Geometry check sheet. Reference: the model listing, model coordinates, mm. Face numbers are marked on the shaded views. A direction names the side the tool comes from. Give positions to 0.01 mm unless a question says otherwise; leave off trailing zeros. Order: outer loops, then holes, each group sorted by start corner. A loop starts at its lowest first (then second) coordinate and runs counter-clockwise, first axis right, second up. Notation, with made-up numbers: M -8,32.5 L 10,32.5 A23 cw 10,48.5 Z; hole C 30,21 d5. An arc over 180 degrees is marked long. Answer as CSV lines item,"result".
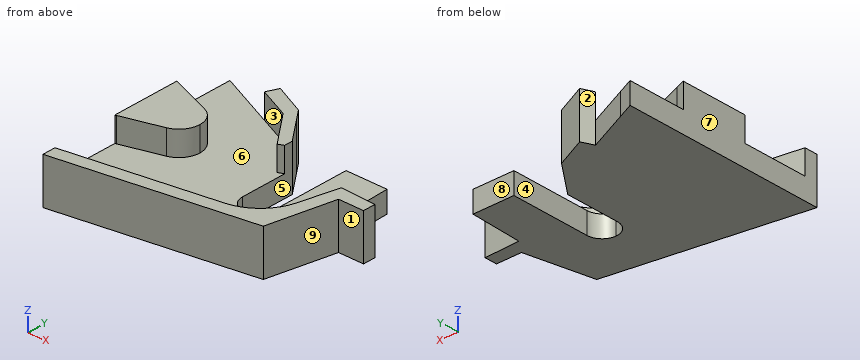
from build123d import *

# Parameters (mm, degrees)
BOSS_EXTRUDE2_DEPTH = 7
BOSS_EXTRUDE3_DEPTH = 15


with BuildPart() as part:
    # Sketch1 → Boss-Extrude2 (new body)
    with BuildSketch(Plane.XY):
        with BuildLine():
            Line((-40.950735345, 0.950710087), (-41.446212302, -3.10814846))
            Line((-41.446212302, -3.10814846), (-41.446212302, -20.792174742))
            Line((-41.446212302, -20.792174742), (-1.475395331, -14.281320254))
            Line((-1.475395331, -14.281320254), (6.869125611, -12.922079544))
            ThreePointArc((6.869125611, -12.922079544), (-10.497186211, -1.975719261), (-2.67291579, 17.003015737))
            Line((-2.67291579, 17.003015737), (-11.698348753, 29.052034329))
            Line((-11.698348753, 29.052034329), (-22.155090004, 33.745741812))
            Line((-22.155090004, 33.745741812), (-36.178915637, 40.040603064))
            Line((-36.178915637, 40.040603064), (-38.38035072, 22.006840878))
            Line((-38.38035072, 22.006840878), (-27.430483413, 17.813364482))
            ThreePointArc((-27.430483413, 17.813364482), (-24.205719333, 15.274219005), (-22.987821209, 11.354641568))
            ThreePointArc((-22.987821209, 11.354641568), (-24.378521993, 7.195004916), (-27.991340604, 4.708206285))
            Line((-27.991340604, 4.708206285), (-40.950735345, 0.950710087))
        make_face()
        Polygon((-41.446212302, 23.180975488), (-38.38035072, 22.006840878), (-36.178915637, 40.040603064), (-41.446212302, 42.4049295), align=None)
        with BuildLine():
            Line((-38.38035072, 22.006840878), (-40.950735345, 0.950710087))
            Line((-40.950735345, 0.950710087), (-27.991340604, 4.708206285))
            ThreePointArc((-27.991340604, 4.708206285), (-30.199701974, 4.44480386), (-32.377484382, 4.895918653))
            ThreePointArc((-32.377484382, 4.895918653), (-36.813821606, 11.650359644), (-31.816627191, 18.00107685))
            ThreePointArc((-31.816627191, 18.00107685), (-29.608265822, 18.264479276), (-27.430483413, 17.813364482))
            Line((-27.430483413, 17.813364482), (-38.38035072, 22.006840878))
        make_face()
        Polygon((-41.446212302, 0.807049614), (-40.950735345, 0.950710087), (-38.38035072, 22.006840878), (-41.446212302, 23.180975488), align=None)
        with BuildLine():
            Line((-32.377484382, 4.895918653), (-29.903983898, 11.354641568))
            Line((-29.903983898, 11.354641568), (-31.816627191, 18.00107685))
            ThreePointArc((-31.816627191, 18.00107685), (-36.813821606, 11.650359644), (-32.377484382, 4.895918653))
        make_face()
        with BuildLine():
            Line((-29.903983898, 11.354641568), (-27.430483413, 17.813364482))
            ThreePointArc((-27.430483413, 17.813364482), (-29.608265822, 18.264479276), (-31.816627191, 18.00107685))
            Line((-31.816627191, 18.00107685), (-29.903983898, 11.354641568))
        make_face()
        with BuildLine():
            ThreePointArc((-32.377484382, 4.895918653), (-30.199701974, 4.44480386), (-27.991340604, 4.708206285))
            Line((-27.991340604, 4.708206285), (-29.903983898, 11.354641568))
            Line((-29.903983898, 11.354641568), (-32.377484382, 4.895918653))
        make_face()
        with BuildLine():
            Line((-29.903983898, 11.354641568), (-27.991340604, 4.708206285))
            ThreePointArc((-27.991340604, 4.708206285), (-24.378521993, 7.195004916), (-22.987821209, 11.354641568))
            ThreePointArc((-22.987821209, 11.354641568), (-24.205719333, 15.274219005), (-27.430483413, 17.813364482))
            Line((-27.430483413, 17.813364482), (-29.903983898, 11.354641568))
        make_face()
        with BuildLine():
            Line((-41.446212302, -20.792174742), (-41.446212302, -25.123400981))
            Line((-41.446212302, -25.123400981), (21.822672825, -14.817519442))
            Line((21.822672825, -14.817519442), (26.489801196, 7.266810726))
            Line((26.489801196, 7.266810726), (34.744303123, 7.266810726))
            Line((34.744303123, 7.266810726), (34.744303123, 11.354641566))
            Line((34.744303123, 11.354641566), (23.2245968, 11.838054321))
            Line((23.2245968, 11.838054321), (20.289273371, -0.393165966))
            ThreePointArc((20.289273371, -0.393165966), (20.186058412, -0.853126065), (20.069286081, -1.309832583))
            ThreePointArc((20.069286081, -1.309832583), (15.501382573, -8.842559665), (7.629856976, -12.798163857))
            ThreePointArc((7.629856976, -12.798163857), (7.250240456, -12.864720887), (6.869125611, -12.922079544))
            Line((6.869125611, -12.922079544), (-1.475395331, -14.281320254))
            Line((-1.475395331, -14.281320254), (-41.446212302, -20.792174742))
        make_face()
        with BuildLine():
            ThreePointArc((-2.67291579, 17.003015737), (-10.497186211, -1.975719261), (6.869125611, -12.922079544))
            Line((6.869125611, -12.922079544), (7.629856976, -12.798163857))
            ThreePointArc((7.629856976, -12.798163857), (15.501382573, -8.842559665), (20.069286081, -1.309832583))
            Line((20.069286081, -1.309832583), (20.289273371, -0.393165966))
            ThreePointArc((20.289273371, -0.393165966), (20.541676305, 1.227855782), (20.626108802, 2.866236051))
            ThreePointArc((20.626108802, 2.866236051), (17.418319473, 12.455992162), (9.086170837, 18.185619879))
            Line((9.086170837, 18.185619879), (9.086170837, 14.654622308))
            Line((9.086170837, 14.654622308), (9.086170837, 9.654622308))
            Line((9.086170837, 9.654622308), (9.086170837, 2.654622308))
            Line((9.086170837, 2.654622308), (9.086170837, -2.345377692))
            Line((9.086170837, -2.345377692), (4.086170856, -2.345377692))
            Line((4.086170856, -2.345377692), (-0.913829163, -2.345377692))
            Line((-0.913829163, -2.345377692), (-0.913829163, 2.654622308))
            Line((-0.913829163, 2.654622308), (-0.913829163, 9.654622308))
            Line((-0.913829163, 9.654622308), (-0.913829163, 14.654622308))
            Line((-0.913829163, 14.654622308), (-2.67291579, 17.003015737))
        make_face()
        with BuildLine():
            Line((20.289273371, -0.393165966), (23.2245968, 11.838054321))
            Line((23.2245968, 11.838054321), (22.586170837, 29.052034329))
            Line((22.586170837, 29.052034329), (9.086170837, 29.052034329))
            Line((9.086170837, 29.052034329), (9.086170837, 18.185619879))
            ThreePointArc((9.086170837, 18.185619879), (17.418319473, 12.455992162), (20.626108802, 2.866236051))
            ThreePointArc((20.626108802, 2.866236051), (20.541676305, 1.227855782), (20.289273371, -0.393165966))
        make_face()
        with BuildLine():
            Line((-11.698348753, 29.052034329), (-2.67291579, 17.003015737))
            ThreePointArc((-2.67291579, 17.003015737), (-1.805237347, 17.421962776), (-0.913829163, 17.787713989))
            Line((-0.913829163, 17.787713989), (-0.913829163, 20.550462038))
            Line((-0.913829163, 20.550462038), (-7.253856265, 29.052034329))
            Line((-7.253856265, 29.052034329), (-10.036820206, 32.783811613))
            Line((-10.036820206, 32.783811613), (-20.38656022, 37.570023616))
            Line((-20.38656022, 37.570023616), (-22.155090004, 33.745741812))
            Line((-22.155090004, 33.745741812), (-11.698348753, 29.052034329))
        make_face()
        Polygon((-41.446212302, 0.807049614), (-41.446212302, -3.10814846), (-40.950735345, 0.950710087), align=None)
        with BuildLine():
            Line((7.629856976, -12.798163857), (6.869125611, -12.922079544))
            ThreePointArc((6.869125611, -12.922079544), (7.250240456, -12.864720887), (7.629856976, -12.798163857))
        make_face()
        with BuildLine():
            Line((20.289273371, -0.393165966), (20.069286081, -1.309832583))
            ThreePointArc((20.069286081, -1.309832583), (20.186058412, -0.853126065), (20.289273371, -0.393165966))
        make_face()
        with BuildLine():
            ThreePointArc((-0.913829163, 17.787713989), (-1.805237347, 17.421962776), (-2.67291579, 17.003015737))
            Line((-2.67291579, 17.003015737), (-0.913829163, 14.654622308))
            Line((-0.913829163, 14.654622308), (-0.913829163, 17.787713989))
        make_face()
        with BuildLine():
            ThreePointArc((4.086170856, -2.345377692), (0.550636938, -0.880911605), (-0.913829163, 2.654622308))
            Line((-0.913829163, 2.654622308), (-0.913829163, -2.345377692))
            Line((-0.913829163, -2.345377692), (4.086170856, -2.345377692))
        make_face()
        with BuildLine():
            Line((9.086170837, -2.345377692), (9.086170837, 2.654622308))
            ThreePointArc((9.086170837, 2.654622308), (7.62170475, -0.880911592), (4.086170856, -2.345377692))
            Line((4.086170856, -2.345377692), (9.086170837, -2.345377692))
        make_face()
    extrude(amount=BOSS_EXTRUDE2_DEPTH)

    # Sketch1_7 → Boss-Extrude3 (add)
    with BuildSketch(Plane.XY):
        with BuildLine():
            Line((-38.38035072, 22.006840878), (-40.950735345, 0.950710087))
            Line((-40.950735345, 0.950710087), (-27.991340604, 4.708206285))
            ThreePointArc((-27.991340604, 4.708206285), (-30.199701974, 4.44480386), (-32.377484382, 4.895918653))
            ThreePointArc((-32.377484382, 4.895918653), (-36.813821606, 11.650359644), (-31.816627191, 18.00107685))
            ThreePointArc((-31.816627191, 18.00107685), (-29.608265822, 18.264479276), (-27.430483413, 17.813364482))
            Line((-27.430483413, 17.813364482), (-38.38035072, 22.006840878))
        make_face()
        with BuildLine():
            Line((-32.377484382, 4.895918653), (-29.903983898, 11.354641568))
            Line((-29.903983898, 11.354641568), (-31.816627191, 18.00107685))
            ThreePointArc((-31.816627191, 18.00107685), (-36.813821606, 11.650359644), (-32.377484382, 4.895918653))
        make_face()
        Polygon((-41.446212302, 0.807049614), (-40.950735345, 0.950710087), (-38.38035072, 22.006840878), (-41.446212302, 23.180975488), align=None)
        with BuildLine():
            Line((-29.903983898, 11.354641568), (-27.991340604, 4.708206285))
            ThreePointArc((-27.991340604, 4.708206285), (-24.378521993, 7.195004916), (-22.987821209, 11.354641568))
            ThreePointArc((-22.987821209, 11.354641568), (-24.205719333, 15.274219005), (-27.430483413, 17.813364482))
            Line((-27.430483413, 17.813364482), (-29.903983898, 11.354641568))
        make_face()
        with BuildLine():
            ThreePointArc((-32.377484382, 4.895918653), (-30.199701974, 4.44480386), (-27.991340604, 4.708206285))
            Line((-27.991340604, 4.708206285), (-29.903983898, 11.354641568))
            Line((-29.903983898, 11.354641568), (-32.377484382, 4.895918653))
        make_face()
        with BuildLine():
            Line((-29.903983898, 11.354641568), (-27.430483413, 17.813364482))
            ThreePointArc((-27.430483413, 17.813364482), (-29.608265822, 18.264479276), (-31.816627191, 18.00107685))
            Line((-31.816627191, 18.00107685), (-29.903983898, 11.354641568))
        make_face()
        with BuildLine():
            Line((-11.698348753, 29.052034329), (-2.67291579, 17.003015737))
            ThreePointArc((-2.67291579, 17.003015737), (-1.805237347, 17.421962776), (-0.913829163, 17.787713989))
            Line((-0.913829163, 17.787713989), (-0.913829163, 20.550462038))
            Line((-0.913829163, 20.550462038), (-7.253856265, 29.052034329))
            Line((-7.253856265, 29.052034329), (-10.036820206, 32.783811613))
            Line((-10.036820206, 32.783811613), (-20.38656022, 37.570023616))
            Line((-20.38656022, 37.570023616), (-22.155090004, 33.745741812))
            Line((-22.155090004, 33.745741812), (-11.698348753, 29.052034329))
        make_face()
        with BuildLine():
            Line((-41.446212302, -20.792174742), (-41.446212302, -25.123400981))
            Line((-41.446212302, -25.123400981), (21.822672825, -14.817519442))
            Line((21.822672825, -14.817519442), (26.489801196, 7.266810726))
            Line((26.489801196, 7.266810726), (34.744303123, 7.266810726))
            Line((34.744303123, 7.266810726), (34.744303123, 11.354641566))
            Line((34.744303123, 11.354641566), (23.2245968, 11.838054321))
            Line((23.2245968, 11.838054321), (20.289273371, -0.393165966))
            ThreePointArc((20.289273371, -0.393165966), (20.186058412, -0.853126065), (20.069286081, -1.309832583))
            ThreePointArc((20.069286081, -1.309832583), (15.501382573, -8.842559665), (7.629856976, -12.798163857))
            ThreePointArc((7.629856976, -12.798163857), (7.250240456, -12.864720887), (6.869125611, -12.922079544))
            Line((6.869125611, -12.922079544), (-1.475395331, -14.281320254))
            Line((-1.475395331, -14.281320254), (-41.446212302, -20.792174742))
        make_face()
    extrude(amount=BOSS_EXTRUDE3_DEPTH)


solid = part.part
(1) Section check A-A on z = 10.25. Enter the section's corners in (x, y).
The answers:
outline,"M -41.45,-25.12 L 21.82,-14.82 L 26.49,7.27 L 34.74,7.27 L 34.74,11.35 L 23.22,11.84 L 20.29,-0.39 A15.94 cw 20.07,-1.31 A15.94 cw 6.87,-12.92 L -41.45,-20.79 Z; M -41.45,0.81 L -27.99,4.71 A6.92 ccw -27.43,17.81 L -41.45,23.18 Z; M -22.16,33.75 L -11.7,29.05 L -2.67,17 A15.94 cw -0.91,17.79 L -0.91,20.55 L -10.04,32.78 L -20.39,37.57 Z"
(2) Section check B-B on x = 10. Enter the section's corners in (y, z).
The answers:
outline,"M -16.74,0 L 29.05,0 L 29.05,7 L -12.16,7 L -12.16,15 L -16.74,15 Z"
(3) Draft check along X on the marked faces 1, 2, 3 and 4. Enter one of: +X half, -X half, draft (parallel to the pull), parting line (faces both ways), or undercut.
The answers:
face 1,"draft"
face 2,"undercut"
face 3,"-X half"
face 4,"undercut"
(4) Section check D-D on x = -15. Enter the section's corners in (y, z), then the cut area to 3 significant figures.
The answers:
outline,"M -20.82,0 L 35.08,0 L 35.08,15 L 30.53,15 L 30.53,7 L -16.48,7 L -16.48,15 L -20.82,15 Z"
area,"462 mm2"
(5) Tool access check on the marked faces 5, 6, 7, 8 and 9. Record the directions out of +Z, -Z, +X, -X, +Y, -Y that give a thin tool (end or side, any length) a straight path to the whole face; none if there is none.
The answers:
face 5,"+Z, -Z, +Y"
face 6,"+Z"
face 7,"+Z, -Z, -X, +Y, -Y"
face 8,"+Z, -Z, +X, +Y"
face 9,"+Z, -Z, +X, -Y"
(6) Section check C-C on y = -5.5. Enter the section's corners in (x, z).
The answers:
outline,"M -41.45,0 L 23.79,0 L 23.79,15 L 18.25,15 L 18.25,7 L -41.45,7 Z"
(7) Material ranges on line 1 (Z direction, x = 22.5, y = 22.5); line 2 (Y direction, x = -12, z = 13.5); line 3 (Y direction, x = -25, z = 7.75), recorded low to high.
The answers:
line 1,"z = 0 to 7"
line 2,"y = -20.33 to -16, 29.19 to 33.69"
line 3,"y = -22.44 to -18.11, 6.48 to 16.23"
(8) Gauge pin test, flat ends, axial feed: P1, Ø2, axis at x = 16.5, z = 4.5, coming from the +Y side; P2, Ø1, axis at x = 4.5, z = 8.5, coming from the +Y side; P3, Ø1, axis at x = -30, z = 6.5, coming from the +Y side. Record the tip position at first contact, or that the pin passes through.
The answers:
P1,"stops at y = 29.05"
P2,"stops at y = -13.23"
P3,"stops at y = 37.49"
